Here's how the part is built. I have some questions about the finished solid (model axes, mm). A direction names the side the tool comes from. Coordinates: 2 decimals unless noted, no trailing zeros. Write each loop counter-clockwise with the first axis right and the second up, starting at its lowest first coordinate (ties: lowest second). Pieces come first, ordered by that corner, then holes.
(1) Please list where these lines run through material, in increasing order: probe 1 along Z at (x, y) = (18, 0); probe 2 along X at (y, z) = (5.4, 0); probe 3 along Z at (x, y) = (7, 0).
(2) Which directions (+Z, -Z, +X, -X, +Y, -Y) give clear straight access to the entire face, cutting with the end or side of a thin tool? Please do faces 3 (the cylindrical face through (15.09, 7.18, 0.07)), 4 (the cylindrical face through (25.697, -1.44, -6.484)), 5 (the cylindrical face through (17.808, -7.803, 0.343)).
(3) For pin 1 Ø3 at (x, y) = (21.5, 2.5) entering from -Z; pin 2 Ø2.5 at (x, z) = (17.5, 0.5) entering from +Y; pin 3 Ø1 at (x, y) = (21, -5.5) entering from +Z; pin 4 Ø3.5 at (y, z) = (-0.5, -0.5) entering from -X, each with a flat end and sliding along its axis, tell me the tip position at first contact or that it passes through.
(4) Imagine slicing it at C-C, the plane z = 0. State how many separate pieces and enclosed holes the cut face has, plus the area to 3 significant figures.
(5) Imagine slicing it at B-B, the plane x = 3.25. List the corners of the cut face in (y, z) for me, plus the area to 3 significant figures.
(6) Thinking about a two-plate mould opening in X: for faces 1 (the cylindrical face through (6.625, -0.991, -4.463)), 2 (the cylindrical face through (2.761, -1.204, -5.424)), which applies, released by +X, released by -X, zero draft, split by the parting line, or undercut?
(7) Imagine slicing it at A-A, the plane x = 19.05. List the corners of the cut face in (y, z) for me.
Autodesk Inventor part; units mm, degrees
ref_plane "c2_XY" through (19.05, 0, 0) normal (0, 0, 1) x (1, 0, 0)
ref_plane "c2_YZ" through (19.05, 0, 0) normal (1, 0, 0) x (0, 1, 0)
ref_plane "c2_ZX" through (19.05, 0, 0) normal (0, 1, 0) x (0, 0, 1)
sketch "Sketch_2" plane through (0, 0, 0) normal (0, 0, 1) x (1, 0, 0)
  line L0 (9.525, 0) -> (0, 0)
  line L1 (0, 0) -> (0, 4.8006)
  line L2 (0, 4.8006) -> (0.7556, 5.5563)
  line L3 (0.7556, 5.5563) -> (4.7111, 5.5563)
  line L4 (4.7111, 5.5563) -> (5.4689, 4.8042)
  arc A0 (5.4689, 4.8042) -> (6.0325, 4.572) centre (6.0325, 5.3721) ccw
  line L5 (6.0325, 4.572) -> (7.2009, 4.572)
  arc A1 (7.2009, 4.572) -> (8.001, 5.3721) centre (7.2009, 5.3721) ccw
  line L6 (8.001, 5.3721) -> (8.001, 5.5309)
  line L7 (8.001, 5.5309) -> (9.525, 5.5309)
  line L8 (9.525, 5.5309) -> (9.525, 0)
  line L9 (9.525, 0) -> (0, 0)
revolve "Revolution1" add sketch "Sketch_2" angle 360 about axis through (9.525, 0, 0) along (1, 0, 0)
thread "Thread1"
sketch "Sketch_3" plane through (0, 0, 0) normal (0, 0, 1) x (1, 0, 0)
  line L0 (29.3624, 0) -> (9.525, 0)
  line L1 (9.525, 0) -> (9.525, 7.0485)
  line L2 (9.525, 7.0485) -> (10.287, 7.8105)
  line L3 (10.287, 7.8105) -> (25.1206, 7.8105)
  line L4 (25.1206, 7.8105) -> (25.3746, 7.5565)
  line L5 (25.3746, 7.5565) -> (25.3746, 6.6421)
  line L6 (25.3746, 6.6421) -> (26.0096, 6.6421)
  line L7 (26.0096, 6.6421) -> (26.6446, 7.2771)
  line L8 (26.6446, 7.2771) -> (28.8544, 7.2771)
  line L9 (28.8544, 7.2771) -> (29.3624, 6.7691)
  line L10 (29.3624, 6.7691) -> (29.3624, 0)
  line L11 (29.3624, 0) -> (9.525, 0)
revolve "Revolution2" add sketch "Sketch_3" angle 360 about axis through (29.3624, 0, 0) along (1, 0, 0)
sketch "Sketch3" plane through (0, 0, 0) normal (-1, 0, 0) x (0, 0, 1)
  point P0 (0, 0)
hole "Hole1" at (0, 0, 0) direction (1, 0, 0) diameter 5.334 depth 29.3624 countersink diameter 6.35 countersink angle 90
sketch "Sketch_13" plane through (0, 0, 0) normal (0, 0, 1) x (1, 0, 0)
  line L0 (19.05, -1.016) -> (19.05, 7.8105)
  line L1 (19.05, 7.8105) -> (23.0124, 7.8105)
  line L2 (23.0124, 7.8105) -> (23.0124, 6.7945)
  line L3 (23.0124, 6.7945) -> (21.463, 6.7945)
  line L4 (21.463, 6.7945) -> (21.0337, 6.3652)
  line L5 (21.0337, 6.3652) -> (21.0337, -1.016)
  line L6 (21.0337, -1.016) -> (19.05, -1.016)
  line L7 (19.05, -1.016) -> (19.05, 7.8105)
revolve "Revolution3" cut sketch "Sketch_13" angle 360 about axis through (19.05, -1.016, 0) along (0, -1, 0)
thread "Thread2"
sketch "Sketch_47" plane through (0, 0, 0) normal (0, 0, 1) x (1, 0, 0)
  line L0 (29.3624, 0) -> (-29.3624, 0)
  line L1 (24.8242, 6.6421) -> (25.1116, 6.6421)
  line L2 (25.1116, 6.6421) -> (26.1958, 7.7263)
  line L3 (26.1958, 7.7263) -> (26.1958, 7.8105)
  line L4 (26.1958, 7.8105) -> (25.9926, 7.8105)
  line L5 (25.9926, 7.8105) -> (24.8242, 6.6421)
revolve "Revolution4" add sketch "Sketch_47" angle 360 about axis through (29.3624, 0, 0) along (1, 0, 0)
ref_plane "c2_XY" through (19.05, 0, 0) normal (0, 0, 1) x (1, 0, 0)
ref_plane "c2_YZ" through (19.05, 0, 0) normal (1, 0, 0) x (0, 1, 0)
ref_plane "c2_ZX" through (19.05, 0, 0) normal (0, 1, 0) x (0, 0, 1)
ref_plane "e2_XY" through (9.525, 0, 0) normal (0, 0, 1) x (1, 0, 0)
ref_plane "e2_YZ" through (9.525, 0, 0) normal (1, 0, 0) x (0, 1, 0)
ref_plane "e2_ZX" through (9.525, 0, 0) normal (0, 1, 0) x (0, 0, 1)
ref_plane "f1_XY" through (8.001, 0, 0) normal (0, 0, 1) x (1, 0, 0)
ref_plane "f1_YZ" through (8.001, 0, 0) normal (1, 0, 0) x (0, 1, 0)
ref_plane "f1_ZX" through (8.001, 0, 0) normal (0, 1, 0) x (0, 0, 1)
ref_plane "f2_XY" through (9.525, 0, 0) normal (0, 0, 1) x (1, 0, 0)
ref_plane "f2_YZ" through (9.525, 0, 0) normal (1, 0, 0) x (0, 1, 0)
ref_plane "f2_ZX" through (9.525, 0, 0) normal (0, 1, 0) x (0, 0, 1)
ref_plane "i1_XY" through (0, 0, -5.5563) normal (0, 1, 0) x (1, 0, 0)
ref_plane "i1_YZ" through (0, 0, -5.5563) normal (1, 0, 0) x (0, 0, -1)
ref_plane "i1_ZX" through (0, 0, -5.5563) normal (0, 0, -1) x (0, 1, 0)
ref_plane "i2_XY" through (0, 0, 5.5563) normal (0, 1, 0) x (1, 0, 0)
ref_plane "i2_YZ" through (0, 0, 5.5563) normal (1, 0, 0) x (0, 0, -1)
ref_plane "i2_ZX" through (0, 0, 5.5563) normal (0, 0, -1) x (0, 1, 0)
ref_plane "l1_XY" through (9.525, 0, -5.5309) normal (0, 1, 0) x (1, 0, 0)
ref_plane "l1_YZ" through (9.525, 0, -5.5309) normal (1, 0, 0) x (0, 0, -1)
ref_plane "l1_ZX" through (9.525, 0, -5.5309) normal (0, 0, -1) x (0, 1, 0)
ref_plane "l2_XY" through (9.525, 0, 5.5309) normal (0, 1, 0) x (1, 0, 0)
ref_plane "l2_YZ" through (9.525, 0, 5.5309) normal (1, 0, 0) x (0, 0, -1)
ref_plane "l2_ZX" through (9.525, 0, 5.5309) normal (0, 0, -1) x (0, 1, 0)
ref_plane "rod_guide_XY" through (0, 0, 0) normal (1, 0, 0) x (0, 0, -1)
ref_plane "rod_guide_YZ" through (0, 0, 0) normal (0, 0, -1) x (0, 1, 0)
ref_plane "rod_guide_ZX" through (0, 0, 0) normal (0, 1, 0) x (1, 0, 0)
ref_plane "to_mounting_bracket_XY" through (9.525, 0, 0) normal (1, 0, 0) x (0, 0, -1)
ref_plane "to_mounting_bracket_YZ" through (9.525, 0, 0) normal (0, 0, -1) x (0, 1, 0)
ref_plane "to_mounting_bracket_ZX" through (9.525, 0, 0) normal (0, 1, 0) x (1, 0, 0)
ref_plane "to_rod_XY" through (-12.7, 0, 0) normal (1, 0, 0) x (0, 0, -1)
ref_plane "to_rod_YZ" through (-12.7, 0, 0) normal (0, 0, -1) x (0, 1, 0)
ref_plane "to_rod_ZX" through (-12.7, 0, 0) normal (0, 1, 0) x (1, 0, 0)
ref_plane "to_tube_XY" through (26.6446, 0, 0) normal (1, 0, 0) x (0, 0, -1)
ref_plane "to_tube_YZ" through (26.6446, 0, 0) normal (0, 0, -1) x (0, 1, 0)
ref_plane "to_tube_ZX" through (26.6446, 0, 0) normal (0, 1, 0) x (1, 0, 0)
properties part number "D-26368----0.5_rod_guide_cyl" material "Steel"
Recorded:
1. probe 1: z = -7.81 to -2.67, 2.67 to 7.81
1. probe 2: x = 0.6 to 4.87, 8 to 17.07, 21.03 to 29.36
1. probe 3: z = -4.57 to -2.67, 2.67 to 4.57
2. face 3: +Y
2. face 4: none
2. face 5: +X, -X
3. pin 1: stops at z = -7.75
3. pin 2: stops at y = 6.79
3. pin 3: stops at z = 6
3. pin 4: passes through
4. separate pieces: 3
4. enclosed holes: 0
4. area: 222 mm2
5. outline: circle Ø11.11 at (0, 0); hole circle Ø5.33 at (0, 0)
5. area: 74.6 mm2
6. face 1: undercut
6. face 2: zero draft
7. outline: (1.78, -1.98) arc R2.67 cw (long way) to (1.78, 1.98) - (6.37, 1.98) - (6.79, 2.41) - (6.79, 3.85) arc R7.81 ccw (long way) to (6.79, -3.85) - (6.79, -2.41) - (6.37, -1.98) - close
